from build123d import *

# Parameters (mm, degrees)
SKETCH7_W           = 100
SKETCH7_H           = 14.5
BOSS_EXTRUDE1_DEPTH = 16.5
SKETCH8_R           = 5
CUT_EXTRUDE2_DEPTH  = 13
CUT_EXTRUDE3_START  = -2
SKETCH9_W           = 27
SKETCH9_H           = 27
CUT_EXTRUDE3_DEPTH  = 2
CUT_EXTRUDE4_DEPTH  = 2
FILLET1_R           = 3
FILLET2_R           = 3


with BuildPart() as part:
    # Sketch7 → Boss-Extrude1 (new body)
    with BuildSketch(Plane(origin=(0, 0, 0), x_dir=(0, 1, 0), z_dir=(0, 0, 1))):
        Rectangle(SKETCH7_W, SKETCH7_H)
    extrude(amount=BOSS_EXTRUDE1_DEPTH)

    # Sketch8 → Cut-Extrude2 (cut)
    with BuildSketch(Plane(origin=(0, 0, 16.5), x_dir=(0, -1, 0), z_dir=(0, 0, 1))):
        with Locations(Location((0, 0, 0), (0, 0, 90))):
            Circle(SKETCH8_R)
    extrude(amount=-CUT_EXTRUDE2_DEPTH, mode=Mode.SUBTRACT)

    # Sketch9 → Cut-Extrude3 (cut)
    with BuildSketch(Plane.XY.offset(16.5).offset(CUT_EXTRUDE3_START)):
        with Locations((0, -31.55)):
            Rectangle(SKETCH9_W, SKETCH9_H)
    cut_extrude3 = extrude(amount=-CUT_EXTRUDE3_DEPTH, mode=Mode.SUBTRACT)

    # Sketch10 → Cut-Extrude4 (cut)
    with BuildSketch(Plane.XY.offset(16.5)):
        with BuildLine():
            Line((0, -24.55), (-7.25, -24.55))
            Line((-7.25, -24.55), (-7.25, -38.55))
            Line((-7.25, -38.55), (0, -38.55))
            ThreePointArc((0, -38.55), (7, -31.55), (0, -24.55))
        make_face()
    cut_extrude4 = extrude(amount=-CUT_EXTRUDE4_DEPTH, mode=Mode.SUBTRACT)

    # Mirror1: Cut-Extrude3 across plane
    add(cut_extrude3.mirror(Plane.ZX), mode=Mode.SUBTRACT)

    # Mirror2: Cut-Extrude4 across plane
    add(cut_extrude4.mirror(Plane.ZX), mode=Mode.SUBTRACT)

    # Fillet1
    fillet1_edges = [part.edges().sort_by_distance(p)[0] for p in [
        (-7.25, 0, 0),
    ]]
    fillet(fillet1_edges, radius=FILLET1_R)

    # Fillet2
    fillet2_edges = [part.edges().sort_by_distance(p)[0] for p in [
        (7.25, 0, 0),
    ]]
    fillet(fillet2_edges, radius=FILLET2_R)


solid = part.part
The listing builds one solid part. Answer for the finished solid, in the listing's coordinates (mm). A direction names the side the tool comes from. Round coordinates to 2 decimals unless told otherwise and drop trailing zeros. Order: outer loops, then holes, each group sorted by start corner. A loop starts at its lowest first (then second) coordinate and runs counter-clockwise, first axis right, second up. Notation, with made-up numbers: (-1, 36.25) -> (47, 36.25) arc R29 cw to (47, 67.25) -> close; hole circle Ø7 at (37, 64). An arc over 180 degrees is marked (long way). Put each result on its own line as item: value.
Q1. Which of the six approach directions +Z, -Z, +X, -X, +Y, -Y give full straight-line access (tool end or side, diameter ignored) to faces 4 (the flat face through (-4, 24.55, 16)), 5 (the cylindrical face through (-1.08, -4.88, 10.09)), 6 (the flat face through (0, -45.05, 14)), 7 (the flat face through (7.25, -1, 10))?
Results list:
face 4: +Z, -X
face 5: +Z
face 6: +X, -X
face 7: +Z, -Z, +X, +Y, -Y
Q2. Section C-C, the plane y = -14.5 is taken. Write down the section's boundary in (x, z), and give its area (3 significant figures).
Results list:
outline: (-7.25, 3) arc R3 ccw to (-4.25, 0) -> (4.25, 0) arc R3 ccw to (7.25, 3) -> (7.25, 16.5) -> (-7.25, 16.5) -> close
area: 235 mm^2
Q3. Section A-A, the plane z = 13.5 is taken. Write down the section's boundary in (x, y).
Results list:
outline: (-7.25, -50) -> (7.25, -50) -> (7.25, -45.05) -> (-7.25, -45.05) -> close; (-7.25, -18.05) -> (7.25, -18.05) -> (7.25, 18.05) -> (-7.25, 18.05) -> close; (-7.25, 45.05) -> (7.25, 45.05) -> (7.25, 50) -> (-7.25, 50) -> close; hole circle Ø10 at (0, 0)
Q4. Consider line 1 along Z through (x, y) = (0.5, -21); line 2 along Y through (x, z) = (0, 11.75); line 3 along Z through (x, y) = (4.5, -13.5). Determine where each line is inside the solid, lowest interval first.
Results list:
line 1: 0 to 12.5, 14.5 to 16.5
line 2: -50 to -5, 5 to 50
line 3: 0.01 to 16.5
Q5. Section D-D, the plane z = 7 is taken. Write down the section's boundary in (x, y).
Results list:
outline: (-7.25, -50) -> (7.25, -50) -> (7.25, 50) -> (-7.25, 50) -> close; hole circle Ø10 at (0, 0)
Q6. Each of these flat-tipped pins is pushed along its axis until it touches: P1, Ø4.5, axis at x = -1, y = -25, coming from the +Z side; P2, Ø4.5, axis at x = -2, y = 32.5, coming from the +Z side. Where does it stop, or does it pass through?
Results list:
P1: z = 16.5
P2: z = 12.5
Q7. Determine the mould class of faces 1 (the flat face through (0, -1, 0)), 2 (the flat face through (5, -25, 14.5)), 3 (the flat face through (-4, 38.55, 16)) for opening direction Z: pulls with the +Z half, pulls with the -Z half, needs draft (parallel to the pull), parting line crosses it, or undercut.
Results list:
face 1: pulls with the -Z half
face 2: undercut
face 3: needs draft
Q8. Section B-B, the plane y = 31.55 is taken. Write down the section's boundary in (x, z), and give its area (3 significant figures).
Results list:
outline: (-7.25, 3) arc R3 ccw to (-4.25, 0) -> (4.25, 0) arc R3 ccw to (7.25, 3) -> (7.25, 12.5) -> (-7.25, 12.5) -> close; (7, 14.5) -> (7.25, 14.5) -> (7.25, 16.5) -> (7, 16.5) -> close
area: 178 mm^2
